Geometry check sheet. Reference: the model listing, model coordinates, mm. A direction names the side the tool comes from. Coordinates: 2 decimals unless noted, no trailing zeros. Write each loop counter-clockwise with the first axis right and the second up, starting at its lowest first coordinate (ties: lowest second). Pieces come first, ordered by that corner, then holes. Notation, with made-up numbers: (2, -2.5) -> (22, -2.5) arc R26 ccw to (22, 19.5) -> close; hole circle Ø4 at (88.5, -31.75). An arc over 180 degrees is marked (long way). One line per question, with ' | ' between items.
```python
from build123d import *

# Parameters (mm, degrees)
SKETCH1_R           = 25.608746635
BOSS_EXTRUDE1_DEPTH = 3
SKETCH2_R           = 8.1
BOSS_EXTRUDE2_DEPTH = 7
SKETCH7_R           = 2.5
CUT_EXTRUDE1_DEPTH  = 10
CIRPATTERN1_COUNT   = 12


with BuildPart() as part:
    # Sketch1 → Boss-Extrude1 (new body)
    with BuildSketch(Plane.XY):
        with Locations((-0.244898521, 0)):
            Circle(SKETCH1_R)
    extrude(amount=BOSS_EXTRUDE1_DEPTH)

    # Sketch2 → Boss-Extrude2 (add)
    with BuildSketch(Plane.XY.offset(3)):
        with BuildLine():
            Line((8.291561976, -12.5), (-8.291561976, -12.5))
            ThreePointArc((-8.291561976, -12.5), (0, 15), (8.291561976, -12.5))
        make_face()
        Circle(SKETCH2_R, mode=Mode.SUBTRACT)
    extrude(amount=BOSS_EXTRUDE2_DEPTH)

    # Sketch4 → CBORE for M3 SHCS1 (revolve, cut)
    with BuildSketch(Plane(origin=(0, 15, 6.5), x_dir=(0, 0, 1), z_dir=(1, 0, 0))):
        Polygon((0, 0), (0, 40.608746635), (1.6, 40.608746635), (1.6, 3), (3.25, 3), (3.25, 0.025), (3.275, 0), align=None)
    revolve(axis=Axis((0, 21.35, 6.5), (0, -1, 0)), mode=Mode.SUBTRACT)

    # Sketch7 → Cut-Extrude1 (cut)
    with BuildSketch(Plane(origin=(0, 0, 0), x_dir=(-1, 0, 0), z_dir=(0, 0, -1))):
        with Locations((0, 22)):
            Circle(SKETCH7_R)
    cut_extrude1 = extrude(amount=-CUT_EXTRUDE1_DEPTH, mode=Mode.SUBTRACT)

    # CirPattern1: Cut-Extrude1 ×12 about axis
    cirpattern1_axis = Axis((0, 0, 0), (0, 0, 1))
    for i in range(1, CIRPATTERN1_COUNT):
        add(cut_extrude1.rotate(cirpattern1_axis, i * 360 / CIRPATTERN1_COUNT), mode=Mode.SUBTRACT)


solid = part.part
```
(1) Material ranges on line 1 (X direction, y = -19, z = 0.75); line 2 (Y direction, x = -1, z = 2); line 3 (Z direction, x = 1.5, y = 19), recorded low to high.
Answers below:
line 1: x = -17.41 to -13.5, -8.5 to 8.5, 13.5 to 16.93 | line 2: y = -25.6 to -24.29, -19.71 to 19.71, 24.29 to 25.6 | line 3: z = 0 to 3
(2) Cross-section at C-C (y = -11). Record the cut outline in (x, z).
Answers below:
outline: (-23.37, 0) -> (-21.55, 0) -> (-21.55, 3) -> (-23.37, 3) -> close; (-16.55, 0) -> (16.55, 0) -> (16.55, 3) -> (10.2, 3) -> (10.2, 10) -> (-10.2, 10) -> (-10.2, 3) -> (-16.55, 3) -> close; (21.55, 0) -> (22.88, 0) -> (22.88, 3) -> (21.55, 3) -> close; hole circle Ø3.2 at (0, 6.5)
(3) Tool access check on faces 4 (the face through (1, 12, 8)), 5 (the face through (17.21, 9.31, 1.48)), 6 (the face through (-1.756, -7.907, 6.451)). Record the directions out of +Z, -Z, +X, -X, +Y, -Y that give a thin tool (end or side, any length) a straight path to the whole face; none if there is none.
Answers below:
face 4: +Y | face 5: +Z, -Z | face 6: +Z
(4) Cross-section at A-A (y = 1.5). Record the cut outline in (x, z), plus the area to 3 significant figures.
Answers below:
outline: (-25.81, 0) -> (-24, 0) -> (-24, 3) -> (-25.81, 3) -> close; (-20, 0) -> (20, 0) -> (20, 3) -> (14.92, 3) -> (14.92, 10) -> (7.96, 10) -> (7.96, 3) -> (-7.96, 3) -> (-7.96, 10) -> (-14.92, 10) -> (-14.92, 3) -> (-20, 3) -> close; (24, 0) -> (25.32, 0) -> (25.32, 3) -> (24, 3) -> close | area: 227 mm²
(5) Cross-section at D-D (x = -11). Record the cut outline in (y, z), plus the area to 3 significant figures.
Answers below:
outline: (-23.24, 0) -> (-21.55, 0) -> (-21.55, 3) -> (-23.24, 3) -> close; (-16.55, 0) -> (16.55, 0) -> (16.55, 3) -> (10.2, 3) -> (10.2, 10) -> (-10.2, 10) -> (-10.2, 3) -> (-16.55, 3) -> close; (21.55, 0) -> (23.24, 0) -> (23.24, 3) -> (21.55, 3) -> close | area: 252 mm²
(6) Draft check along Y on faces 1 (the face through (2, -12.5, 6)), 2 (the face through (4, 8, 10)), 3 (the face through (24.48, -0.33, 1.48)). Enter one of: pulls with the +Y half, pulls with the -Y half, needs draft (parallel to the pull), parting line crosses it, or undercut.
Answers below:
face 1: pulls with the -Y half | face 2: needs draft | face 3: undercut
(7) Depth check by flat-ended pin: P1, Ø6.5, axis at x = 11, y = 19.05, coming from the -Z side; P2, Ø3.5, axis at x = -2.5, z = 5.5, coming from the -Y side; P3, Ø3, axis at x = 10.5, z = 9, coming from the -Y side; P4, Ø6, axis at x = 22, y = 0, coming from the +Z side. Enter the tip coordinate at first touch or a pass-through.
Answers below:
P1: stops at z = 0 | P2: stops at y = -12.5 | P3: stops at y = -12 | P4: stops at z = 3
(8) Cross-section at B-B (z = 5.5). Record the cut outline in (x, y).
Answers below:
outline: (-8.29, -12.5) -> (-1.25, -12.5) -> (-1.25, -8) arc R8.1 cw to (-1.25, 8) -> (-1.25, 12) -> (-3.09, 12) -> (-3.09, 14.68) arc R15 ccw to start; (1.25, -12.5) -> (8.29, -12.5) arc R15 ccw to (3.09, 14.68) -> (3.09, 12) -> (1.25, 12) -> (1.25, 8) arc R8.1 cw to (1.25, -8) -> close
